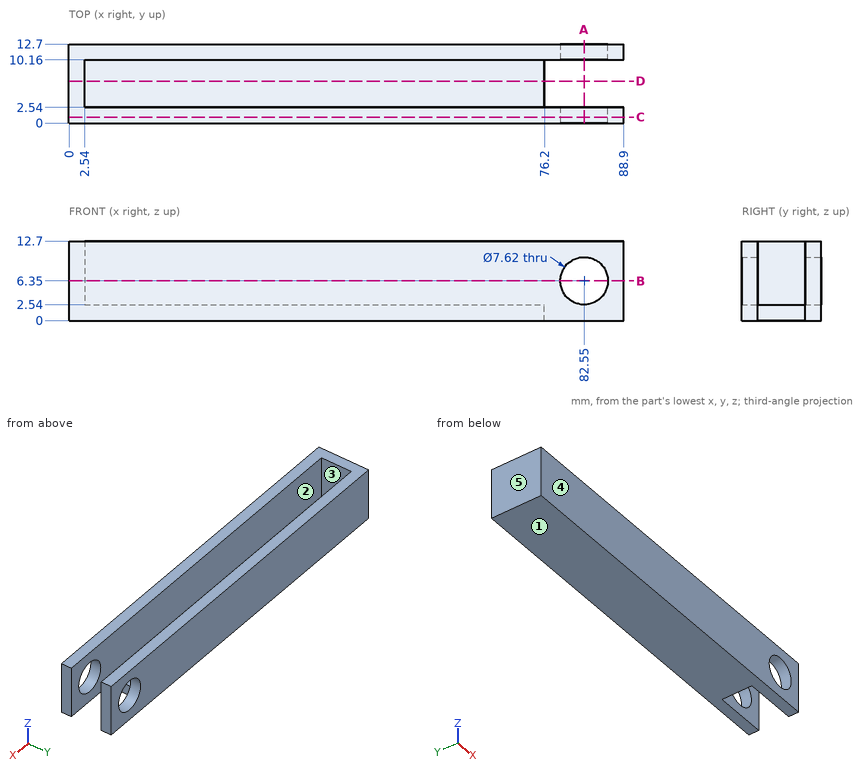
Study the drawing (mm; zero at the part's minimum x, y, z) and answer. A direction names the side the tool comes from. Give positions to 0.01 mm unless a question says otherwise; leave off trailing zeros. Loops run counter-clockwise (first coordinate to the right, second up) from the corner with the lowest first, then second, coordinate; pieces in that order, holes last. Notation, with made-up numbers: (-21, -16.5) - (4, -16.5) arc R28 ccw to (4, 21.5) - close; hole circle Ø5 at (-31, 38). An arc over 180 degrees is marked (long way). One line per question, with ' | ' between items.
(1) This flat-tipped pin is pushed along its axis until it touches: pin 1 Ø2 at (y, z) = (4.5, 1) entering from +X. Where does it stop, or does it pass through?
Recorded:
pin 1: stops at x = 76.2
(2) The part is cut by section C-C (y = 1). Write down the section's boundary in (x, z).
Recorded:
outline: (0, 0) - (88.9, 0) - (88.9, 12.7) - (0, 12.7) - close; hole circle Ø7.62 at (82.55, 6.35)
(3) Straight lines are drawn through the part: probe 1 along Y at (x, z) = (17.5, 6.5); probe 2 along X at (y, z) = (7, 4.75). For each, find the intervals that lie inside material, in ascending order.
Recorded:
probe 1: y = 0 to 2.54, 10.16 to 12.7 | probe 2: x = 0 to 2.54
(4) The part is cut by section B-B (z = 6.35). Write down the section's boundary in (x, y).
Recorded:
outline: (0, 0) - (78.74, 0) - (78.74, 2.54) - (2.54, 2.54) - (2.54, 10.16) - (78.74, 10.16) - (78.74, 12.7) - (0, 12.7) - close; (86.36, 0) - (88.9, 0) - (88.9, 2.54) - (86.36, 2.54) - close; (86.36, 10.16) - (88.9, 10.16) - (88.9, 12.7) - (86.36, 12.7) - close
(5) A tool of negligible diameter and unlimited length cuts with its end or side. For the marked faces 1 and 2, from which of +Z, -Z, +X, -X, +Y, -Y can it reach the whole face along a straight path? Write none if from no direction.
Recorded:
face 1: -Z, +X, -X, +Y, -Y | face 2: +Z, +X
(6) The part is cut by section A-A (x = 82.55). Write down the section's boundary in (y, z).
Recorded:
outline: (0, 0) - (2.54, 0) - (2.54, 2.54) - (0, 2.54) - close; (0, 10.16) - (2.54, 10.16) - (2.54, 12.7) - (0, 12.7) - close; (10.16, 0) - (12.7, 0) - (12.7, 2.54) - (10.16, 2.54) - close; (10.16, 10.16) - (12.7, 10.16) - (12.7, 12.7) - (10.16, 12.7) - close
(7) The part is cut by section D-D (y = 6.75). Write down the section's boundary in (x, z), then the cut area to 3 significant figures.
Recorded:
outline: (0, 0) - (76.2, 0) - (76.2, 2.54) - (2.54, 2.54) - (2.54, 12.7) - (0, 12.7) - close | area: 219 mm²
(8) The mould has two halves that part along Y. Classify the marked faces 3, 4 and 5: +Y half, -Y half, draft (parallel to the pull), parting line (faces both ways), or undercut.
Recorded:
face 3: undercut | face 4: -Y half | face 5: draft
